from build123d import *

# Parameters (mm, degrees)
F0_W     = 116.736240685
F0_H     = 45.7762465812
F1_DEPTH = 25.4
F3_DEPTH = 20.32


with BuildPart() as f1:
    # F0 (on Right) → F1 (new body)
    with BuildSketch(Plane.YZ):
        Polygon((-60.9279610217, -47.761421484), (-60.9279610217, -60.461421484), (66.0720389783, -60.461421484), (66.0720389783, -45.2970974147), (66.0720389783, -42.7577458322), (66.0720389783, -40.2231365442), (66.0720389783, -37.6602597535), (66.0720389783, -35.1163968444), (66.0720389783, -32.5725339353), (66.0720389783, -30.0129074603), (66.0720389783, -27.4480152875), (66.0720389783, -25.4), (66.0720389783, -22.361421484), (63.5299555494, -22.8698381698), (63.5299555494, -56.7358210683), (-58.5926286876, -56.7358210683), (-58.5926286876, -47.2943550172), (-59.6095568016, -47.49774064), align=None)
        Polygon((-60.9279610217, 3.0077947435), (-60.9279610217, -47.761421484), (-59.6095568016, -47.49774064), (-59.6095568016, -16.7404655367), (-59.6095568016, 3.0077947435), align=None)
        Polygon((-60.9279610217, 53.8077947435), (-60.9279610217, 3.0077947435), (-59.6095568016, 3.0077947435), (-59.6095568016, 88.458865881), (-55.3284734488, 88.458865881), (-55.3284734488, 54.3211102486), (-55.3284734488, 3.0077947435), (63.5299555494, 3.0077947435), (66.0720389783, 3.0077947435), (66.0720389783, 53.838578516), (-53.3079610217, 53.838578516), (-53.3079610217, 91.938578516), (-60.9279610217, 91.938578516), align=None)
        with Locations((4.933912307, 28.6751843523)):
            Rectangle(F0_W, F0_H, mode=Mode.SUBTRACT)
        Polygon((66.0720389783, 3.0077947435), (63.5299555494, 3.0077947435), (63.5299555494, -22.8698381698), (66.0720389783, -22.361421484), align=None)
        Polygon((-58.2911525815, -47.234059796), (-58.5926286876, -47.2943550172), (-58.5926286876, -56.7358210683), (63.5299555494, -56.7358210683), (63.5299555494, -22.8698381698), (54.6891463984, -24.638), (54.6891463984, 0), (50.8791463984, 0), (50.8791463984, -25.4), (44.4574505091, -26.6843391779), (44.4574505091, 0), (40.6390699608, 0), (40.6390699608, -27.4480152875), (31.6170305014, -29.2524231794), (31.6170305014, 0), (27.8146090967, 0), (27.8146090967, -30.0129074603), (18.8264767218, -31.8105339353), (18.8264767218, 0), (15.0164767218, 0), (15.0164767218, -32.5725339353), (6.3523404126, -34.3053611972), (6.3820375505, -0.0032985204), (2.5720389783, 0), (2.5720389783, -35.061421484), (-5.1686692631, -36.6095631323), (-5.1686692631, -0.0032985204), (-8.9786678353, 0), (-9.1092809997, -37.3976854796), (-19.0416296813, -39.3841552159), (-19.0416296813, -0.0133065219), (-22.8516064445, 0), (-22.8516064445, -40.1461505686), (-30.3492701047, -41.6456833006), (-30.3492701047, 0), (-34.1592701047, 0), (-34.1592701047, -42.4076833006), (-41.7353913358, -43.9229075468), (-41.7353913358, -0.0208968543), (-45.5453340285, 0), (-45.5453340285, -44.6848960854), (-54.4811525815, -46.472059796), (-54.4811525815, 0), (-58.2911525815, 0), align=None)
    extrude(amount=F1_DEPTH)

    # F2 (on face) → F3 (cut)
    with BuildSketch(Plane(origin=(0, 0, 0), x_dir=(0, -1, 0), z_dir=(-1, 0, 0))):
        Polygon((-66.0720389783, -22.361421484), (-66.0720389783, -22.8698381698), (-66.0720389783, -60.461421484), (60.9279610217, -60.461421484), (60.9279610217, -47.49774064), (59.6095568016, -47.365900218), (59.6095568016, -47.49774064), (58.2911525815, -47.234059796), (58.2911525815, 0), (54.4811525815, 0), (54.4811525815, -46.472059796), (45.5453340285, -44.6848960854), (45.5453340285, 0), (41.7353913358, -0.0208968543), (41.7353913358, -43.9229075468), (34.1592701047, -42.4076833006), (34.1592701047, 0), (30.3492701047, 0), (30.3492701047, -41.6456833006), (22.8516064445, -40.1461505686), (22.8516064445, 0), (19.0416296813, -0.0133065219), (19.0416296813, -39.3841552159), (9.1092809997, -37.3976854796), (8.9786678353, 0), (5.1686692631, -0.0032985204), (5.1686692631, -36.6095631323), (-2.5720389783, -35.061421484), (-2.5720389783, 0), (-6.3820375505, -0.0032985204), (-6.3523404126, -34.3053611972), (-15.0164767218, -32.5725339353), (-15.0164767218, 0), (-18.8264767218, 0), (-18.8264767218, -31.8105339353), (-27.8146090967, -30.0129074603), (-27.8146090967, 0), (-31.6170305014, 0), (-31.6170305014, -29.2524231794), (-40.6390699608, -27.4480152875), (-40.6390699608, 0), (-44.4574505091, 0), (-44.4574505091, -26.6843391779), (-50.8791463984, -25.4), (-50.8791463984, 0), (-54.6891463984, 0), (-54.6891463984, -24.638), (-63.5299555494, -22.8698381698), align=None)
    extrude(amount=-F3_DEPTH, mode=Mode.SUBTRACT)


solid = f1.part
The model under review builds one solid part; all positions refer to its coordinate system, in mm. A direction names the side the tool comes from. Round coordinates to 2 decimals unless told otherwise and drop trailing zeros. Loops run counter-clockwise (first coordinate to the right, second up) from the corner with the lowest first, then second, coordinate; pieces in that order, holes last. Notation, with made-up numbers: M 78.5,64 L 85.5,64 A22 cw 85.5,75 Z; hole C 70,57.5 d3. An arc over 180 degrees is marked long. Answer as a JSON object with one key per item and string values.
Item 1: We need section A-A, the plane z = 80. State the section outline as (x, y) points, and give its area (3 significant figures).
Check sheet entries:
{"outline": "M 0,-60.93 L 25.4,-60.93 L 25.4,-59.61 L 0,-59.61 Z; M 0,-55.33 L 25.4,-55.33 L 25.4,-53.31 L 0,-53.31 Z", "area": "84.8 mm2"}
Item 2: Clearance check with flat-ended pins moving along their axes: P1, Ø10, axis at x = 12.5, y = 38, coming from the +Z side; P2, Ø7.5, axis at x = 14, y = 32.5, coming from the -Z side; P3, Ø6, axis at y = 33.5, z = -0.5, coming from the -X side. State where each tip first meets the part, or that it passes through.
Check sheet entries:
{"P1": "z = 53.84", "P2": "z = 3.01", "P3": "x = 20.32"}
Item 3: We need section C-C, the plane z = 8.5. State the section outline as (x, y) points, and give its area (3 significant figures).
Check sheet entries:
{"outline": "M 0,-60.93 L 25.4,-60.93 L 25.4,-59.61 L 0,-59.61 Z; M 0,-55.33 L 25.4,-55.33 L 25.4,-53.43 L 0,-53.43 Z; M 0,63.3 L 25.4,63.3 L 25.4,66.07 L 0,66.07 Z", "area": "152 mm2"}
Item 4: We need section D-D, the plane y = -39.5. State the section outline as (x, z) points.
Check sheet entries:
{"outline": "M 0,3.01 L 25.4,3.01 L 25.4,5.79 L 0,5.79 Z; M 0,51.56 L 25.4,51.56 L 25.4,53.84 L 0,53.84 Z; M 20.32,-60.46 L 25.4,-60.46 L 25.4,-43.48 L 20.32,-43.48 Z"}
Item 5: For line 1 along Z through (x, y) = (23, -31.5); line 2 along Y through (x, z) = (7.5, 7.5); line 3 along Y through (x, z) = (14, -15), list the stretches that pass through material, from the lowest coordinate up.
Check sheet entries:
{"line 1": "-60.46 to 0, 3.01 to 5.79, 51.56 to 53.84", "line 2": "-60.93 to -59.61, -55.33 to -53.43, 63.3 to 66.07", "line 3": "-60.93 to -59.61, 63.53 to 66.07"}
Item 6: Tool access review of faces 5 (the face through (13, -57, 91.939)), 6 (the face through (22.824, 47.713, -26.033)): name each direction out of +Z, -Z, +X, -X, +Y, -Y from which nothing blocks a thin tool from reaching the whole face with its end or side.
Check sheet entries:
{"face 5": "+Z, +X, -X, +Y, -Y", "face 6": "+X, -X"}
Item 7: The part is to be moulded in two halves that separate along Z. For faces 1 (the face through (13, 63.53, -10)), 2 (the face through (20.32, 18, -37)), 3 (the face through (23, 27.815, -15)), 4 (the face through (23, 2, -60.461)), say which applies: +Z half, -Z half, draft (parallel to the pull), parting line (faces both ways), or undercut.
Check sheet entries:
{"face 1": "undercut", "face 2": "draft", "face 3": "undercut", "face 4": "-Z half"}
Item 8: We need section B-B, the plane x = 9.25. State the section outline as (y, z) points.
Check sheet entries:
{"outline": "M -60.93,-47.5 L -59.61,-47.37 L -59.61,88.46 L -55.33,88.46 L -55.33,3.01 L 63.53,3.01 L 63.53,-22.87 L 66.07,-22.36 L 66.07,53.84 L -53.31,53.84 L -53.31,91.94 L -60.93,91.94 Z; hole M -53.43,5.79 L 63.3,5.79 L 63.3,51.56 L -53.43,51.56 Z"}
